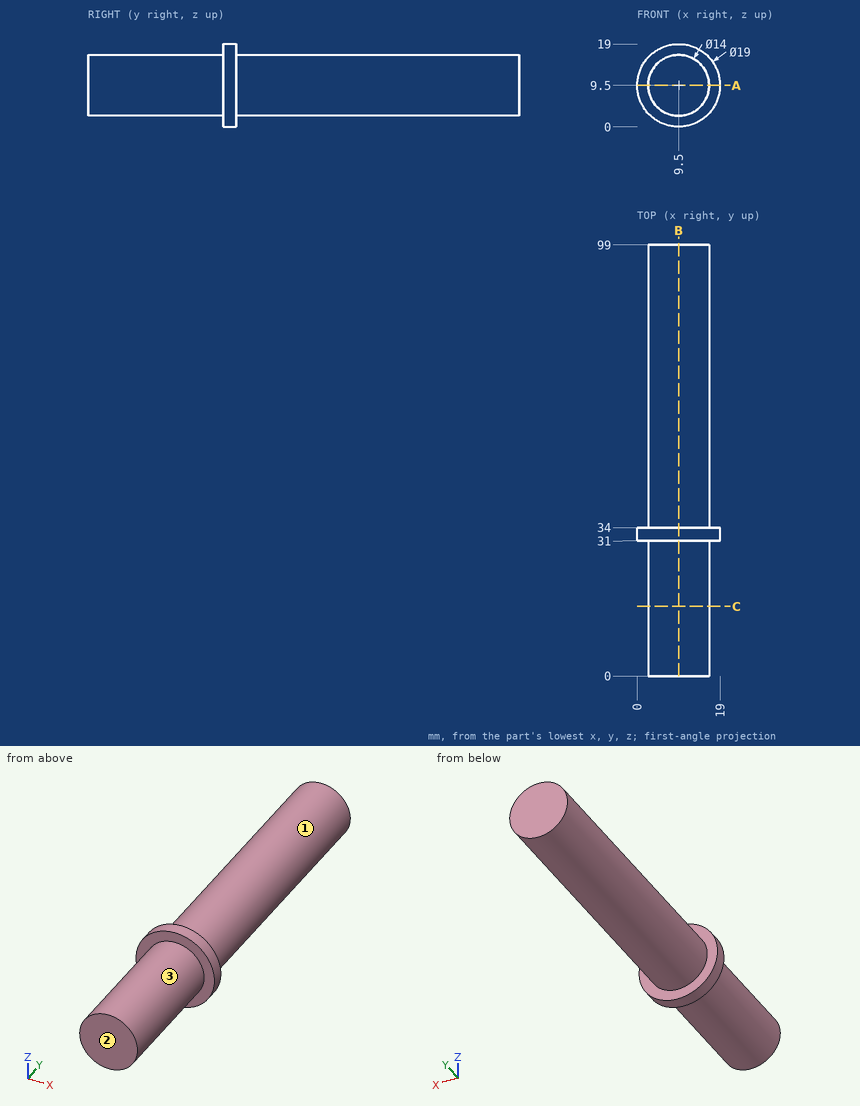
Can you work these out from the drawing? Everything is in mm from the part's minimum corner. A direction names the side the tool comes from. Round coordinates to 2 decimals unless told otherwise and drop trailing zeros. Order: outer loops, then holes, each group sorted by start corner. A loop starts at its lowest first (then second) coordinate and runs counter-clockwise, first axis right, second up.
(1) If we section it at B-B (x = 9.5): Please give me the cut outline in (y, z).
Results are:
outline: (0, 2.5) - (31, 2.5) - (31, 0) - (34, 0) - (34, 2.5) - (99, 2.5) - (99, 16.5) - (34, 16.5) - (34, 19) - (31, 19) - (31, 16.5) - (0, 16.5) - close
(2) If we section it at C-C (y = 16): Please give me the cut outline in (x, z).
Results are:
outline: circle Ø14 at (9.5, 9.5)
(3) If I drill on L1, parallel to Y at x = 15.5, z = 16; L2, parallel to X at y = 53.5, z = 14.25; L3, parallel to Z at x = 12.5, y = 89.5, over which ranges is the centre line in solid material (lowest first)?
Results are:
L1: y = 31 to 34
L2: x = 4.36 to 14.64
L3: z = 3.18 to 15.82
(4) I'm going to push flat-ended pins straight in: pin 1 (1 mm diameter, centred on x = 12, y = 28, fed in from -Z); pin 2 (3 mm diameter, centred on y = 56, z = 8.5, fed in from +X); pin 3 (1.5 mm diameter, centred on x = 5.5, y = 44, fed in from -Z). Where does each tip first touch, or does it pass through?
Results are:
pin 1: stops at z = 2.79
pin 2: stops at x = 16.5
pin 3: stops at z = 3.3
(5) If we section it at A-A (z = 9.5): Please give me the cut outline in (x, y).
Results are:
outline: (0, 31) - (2.5, 31) - (2.5, 0) - (16.5, 0) - (16.5, 31) - (19, 31) - (19, 34) - (16.5, 34) - (16.5, 99) - (2.5, 99) - (2.5, 34) - (0, 34) - close
(6) On a 3-axis mill with a long thin cutter (end or side, diameter ignored), from which of +Z, -Z, +X, -X, +Y, -Y can I reach the whole of each face in a straight line? I mean the marked faces 1, 2 and 3. Say none if no direction works.
Results are:
face 1: +Y
face 2: +Z, -Z, +X, -X, -Y
face 3: -Y
